from build123d import *

# Parameters (mm, degrees)
SKETCH_1_R           = 2
SKETCH_1_R_2         = 1.4
EXTRUDE_1_DEPTH      = 10
SKETCH_2_R           = 1.4
EXTRUDE_2_DEPTH      = 10
EXTRUDE_3_DEPTH      = 2
EXTRUDE_3_DEPTH_BACK = 12
SKETCH_3_R           = 1.4


with BuildPart() as part:
    # 草图1 → 凸台-拉伸1 (new body)
    with BuildSketch(Plane.XY):
        Circle(SKETCH_1_R)
        Circle(SKETCH_1_R_2, mode=Mode.SUBTRACT)
    extrude(amount=EXTRUDE_1_DEPTH)

    # 草图2 → 凸台-拉伸2 (add)
    with BuildSketch(Plane(origin=(0, 0, 0), x_dir=(-1, 0, 0), z_dir=(0, 0, -1))):
        Circle(SKETCH_2_R)
    extrude(amount=-EXTRUDE_2_DEPTH)

    # 草图3 → 凸台-拉伸3 (add, two sides: drawn at the far end of the back side and taken through both)
    with BuildSketch(Plane(origin=(0, 0, 0), x_dir=(-1, 0, 0), z_dir=(0, 0, -1)).offset(-EXTRUDE_3_DEPTH_BACK)):
        Circle(SKETCH_3_R)
    extrude(amount=EXTRUDE_3_DEPTH + EXTRUDE_3_DEPTH_BACK)


solid = part.part
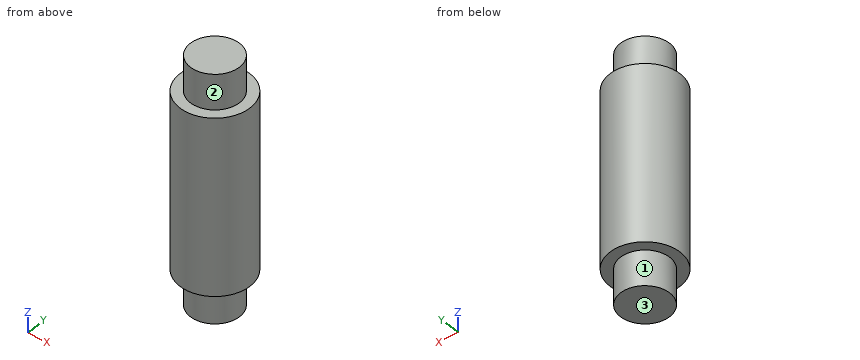
Design review of the part built by this model. Coordinates are the model's own, in mm. Face numbers are marked on the shaded views. A direction names the side the tool comes from. Round coordinates to 2 decimals unless told otherwise and drop trailing zeros. Write each loop counter-clockwise with the first axis right and the second up, starting at its lowest first coordinate (ties: lowest second). Pieces come first, ordered by that corner, then holes. Notation, with made-up numbers: (-15, 43.25) - (-3, 43.25) arc R11 ccw to (-3, 53.25) - close; hole circle Ø7 at (23.25, -31.75). An arc over 180 degrees is marked (long way). Use a Markdown table: item, result. Add a question column.
1. For the marked faces 1, 2 and 3, list the 3-axis set-ups (+Z, -Z, +X, -X, +Y, -Y) from which the entire face can be reached by the end or side of a thin tool; tool diameter is ignored.
2. Wall thickness on probe 1 along Z at (x, y) = (-1.4, -0.4); probe 2 along Y at (x, z) = (0.1, 9.25); probe 3 along Y at (x, z) = (-1.8, 3.5): over which ranges is each line inside the solid? List them lowest first.
3. Clearance check with a flat-ended pin moving along its axis: pin 1 (1.5 mm diameter, centred on y = -1.5, z = 10, fed in from +X). State where the tip first meets the part, or that it passes through.
4. We need section C-C (z = -0.25). State the section outline as (x, y) points.
5. We need section B-B (y = -0.9). State the section outline as (x, z) points.
6. We need section A-A (x = 0). State the section outline as (y, z) points.
7. We need section D-D (z = 7.75). State the section outline as (x, y) points, then the cut area to 3 significant figures.
Output:
| question | item | result |
|---|---|---|
| 1 | face 1 | -Z |
| 1 | face 2 | +Z |
| 1 | face 3 | -Z, +X, -X, +Y, -Y |
| 2 | probe 1 | z = 0 to 10 |
| 2 | probe 2 | y = -2 to 2 |
| 2 | probe 3 | y = -0.87 to 0.87 |
| 3 | pin 1 | stops at x = 1.85 |
| 4 | outline | circle Ø2.8 at (0, 0) |
| 5 | outline | (-1.79, 0) - (-1.07, 0) - (-1.07, -2) - (1.07, -2) - (1.07, 0) - (1.79, 0) - (1.79, 10) - (1.07, 10) - (1.07, 12) - (-1.07, 12) - (-1.07, 10) - (-1.79, 10) - close |
| 6 | outline | (-2, 0) - (-1.4, 0) - (-1.4, -2) - (1.4, -2) - (1.4, 0) - (2, 0) - (2, 10) - (1.4, 10) - (1.4, 12) - (-1.4, 12) - (-1.4, 10) - (-2, 10) - close |
| 7 | outline | circle Ø4 at (0, 0) |
| 7 | area | 12.6 mm2 |
